Work out the finished part from the listing and answer in its coordinate system (mm). Face numbers are marked on the shaded views. A direction names the side the tool comes from. Give positions to 0.01 mm unless a question says otherwise; leave off trailing zeros. Write each loop counter-clockwise with the first axis right and the second up, starting at its lowest first coordinate (ties: lowest second). Pieces come first, ordered by that corner, then holes. Notation, with made-up numbers: (54.5, 66.5) - (90.5, 66.5) arc R15 cw to (90.5, 75.5) - close; hole circle Ø2 at (0, 74). An arc over 180 degrees is marked (long way). Write item = value, one per line.
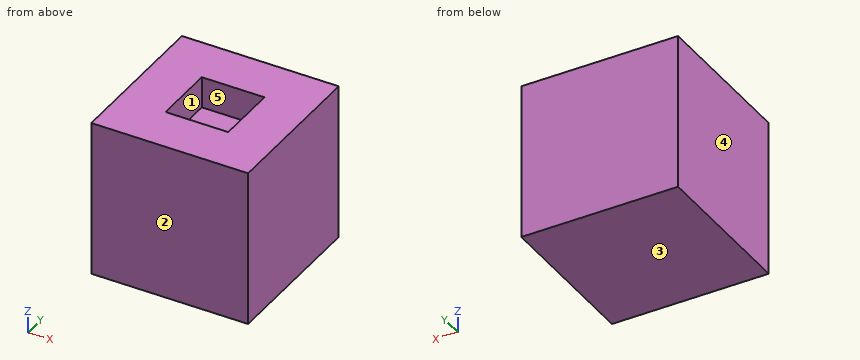
from build123d import *

# Parameters (mm, degrees)
F0_W     = 127
F0_H     = 127
F1_DEPTH = 63.5
F2_W     = 50.8
F2_H     = 50.8
F3_DEPTH = 25.4


with BuildPart() as f1:
    # F0 (on Front) → F1 (new body, symmetric)
    with BuildSketch(Plane.XZ):
        Rectangle(F0_W, F0_H)
    extrude(amount=F1_DEPTH, both=True)

    # F2 (on face) → F3 (cut)
    with BuildSketch(Plane.XY.offset(63.5)):
        Rectangle(F2_W, F2_H)
    extrude(amount=-F3_DEPTH, mode=Mode.SUBTRACT)


solid = f1.part
1. For a pull along Y with two mould halves and no side action, classify the marked faces 1, 2 and 3 as pulls with the +Y half, pulls with the -Y half, needs draft (parallel to the pull), parting line crosses it, or undercut.
Solution:
face_1 = undercut
face_2 = pulls with the -Y half
face_3 = needs draft
2. A tool of negligible diameter and unlimited length cuts with its end or side. For the marked faces 4 and 5, from which of +Z, -Z, +X, -X, +Y, -Y can it reach the whole face along a straight path? Write none if from no direction.
Solution:
face_4 = +Z, -Z, -X, +Y, -Y
face_5 = +Z
3. Find section B-B, the plane y = -10.5. Give the vertices of the cut face in (x, z).
Solution:
outline = (-63.5, -63.5) - (63.5, -63.5) - (63.5, 63.5) - (25.4, 63.5) - (25.4, 38.1) - (-25.4, 38.1) - (-25.4, 63.5) - (-63.5, 63.5) - close
4. A straight line is drawn through the part: line 1 (Y direction, x = 25, z = 45.5). Find the intervals that lie inside material, in ascending order.
Solution:
line_1 = -63.5 to -25.4, 25.4 to 63.5
5. Given pin 1 (15 mm diameter, centred on x = 8.5, y = -5, fed in from +Z), flat-ended and moving along its own axis, determine where the tip first touches the part or whether it passes through.
Solution:
pin_1 = 38.1
6. Find section A-A, the plane z = 46.5. Give the vertices of the cut face in (x, y), then the cut area to 3 significant figures.
Solution:
outline = (-63.5, -63.5) - (63.5, -63.5) - (63.5, 63.5) - (-63.5, 63.5) - close; hole (-25.4, -25.4) - (25.4, -25.4) - (25.4, 25.4) - (-25.4, 25.4) - close
area = 13,500 mm^2
